from build123d import *

# Parameters (mm, degrees)
BOSS_EXTRUDE1_DEPTH                              = 10
CBORE_FOR_1_4_SOCKET_HEAD_CAP_SCREW1_D           = 7.14248
CBORE_FOR_1_4_SOCKET_HEAD_CAP_SCREW1_CBORE_D     = 11.1125
CBORE_FOR_1_4_SOCKET_HEAD_CAP_SCREW1_CBORE_DEPTH = 6.35
SKETCH5_W                                        = 12.7
SKETCH5_H                                        = 2
BOSS_EXTRUDE2_DEPTH                              = 14
CUT_EXTRUDE1_DEPTH                               = 10
SKETCH7_R                                        = 4
CUT_EXTRUDE2_DEPTH                               = 10


with BuildPart() as part:
    # Sketch1 → Boss-Extrude1 (new body)
    with BuildSketch(Plane(origin=(0, 0, 0), x_dir=(1, 0, 0), z_dir=(0, 1, 0))):
        with BuildLine():
            Line((6.35, 12.7), (6.35, -12.7))
            ThreePointArc((6.35, -12.7), (0, -19.05), (-6.35, -12.7))
            Line((-6.35, -12.7), (-6.35, 12.7))
            ThreePointArc((-6.35, 12.7), (0, 19.05), (6.35, 12.7))
        make_face()
    extrude(amount=BOSS_EXTRUDE1_DEPTH)

    # CBORE for 1/4 Socket Head Cap Screw1 (through all)
    with Locations(Plane(origin=(0, 10, 0), x_dir=(1, 0, 0), z_dir=(0, 1, 0))):
        with Locations((0, -12.7)):
            CounterBoreHole(CBORE_FOR_1_4_SOCKET_HEAD_CAP_SCREW1_D / 2, CBORE_FOR_1_4_SOCKET_HEAD_CAP_SCREW1_CBORE_D / 2, CBORE_FOR_1_4_SOCKET_HEAD_CAP_SCREW1_CBORE_DEPTH)

    # Sketch5 → Boss-Extrude2 (add)
    with BuildSketch(Plane(origin=(0, 10, 0), x_dir=(1, 0, 0), z_dir=(0, 1, 0))):
        Rectangle(SKETCH5_W, SKETCH5_H)
    extrude(amount=BOSS_EXTRUDE2_DEPTH)

    # Sketch6 → Cut-Extrude1 (cut)
    with BuildSketch(Plane.XY.offset(1)):
        with BuildLine():
            Line((-6.35, 24), (-6.35, 17.65))
            ThreePointArc((-6.35, 17.65), (-4.490128051, 22.14012807), (2.8e-08, 24))
            Line((2.8e-08, 24), (-6.35, 24))
        make_face()
        with BuildLine():
            Line((6.35, 24), (2.8e-08, 24))
            ThreePointArc((2.8e-08, 24), (4.49012807, 22.140128051), (6.35, 17.65))
            Line((6.35, 17.65), (6.35, 24))
        make_face()
    extrude(amount=-CUT_EXTRUDE1_DEPTH, mode=Mode.SUBTRACT)

    # Sketch7 → Cut-Extrude2 (cut)
    with BuildSketch(Plane.XY.offset(1)):
        with Locations((0, 17.65)):
            Circle(SKETCH7_R)
    extrude(amount=-CUT_EXTRUDE2_DEPTH, mode=Mode.SUBTRACT)


solid = part.part
The listing builds one solid part. Answer for the finished solid, in the listing's coordinates (mm). A direction names the side the tool comes from. Coordinates: 2 decimals unless noted, no trailing zeros. Loops run counter-clockwise (first coordinate to the right, second up) from the corner with the lowest first, then second, coordinate; pieces in that order, holes last. Notation, with made-up numbers: (-24.75, -8) -> (33.25, -8) arc R22 ccw to (33.25, 11) -> close; hole circle Ø11 at (69.5, 44.5). An arc over 180 degrees is marked (long way). Write item = value, one per line. Start each with the question number.
1) A cutting plane is placed at A-A (x = -2). Give the vertices of the cut face in (y, z).
2) A cutting plane is placed at C-C (y = 16.5). Give the vertices of the cut face in (x, z).
3) Given pin 1 Ø6.5 at (x, z) = (0, 12.7) entering from -Y; pin 2 Ø6 at (x, y) = (3.5, 6) entering from +Z; pin 3 Ø6 at (x, y) = (-3.5, 14) entering from -Z; pin 4 Ø2 at (x, z) = (-0.5, -5.5) entering from -Y, each flat-ended and moving along its own axis, determine where each tip first touches the part or whether it passes through.
4) Straight lines are drawn through the part: line 1 (Z direction, x = 0, y = 0.9); line 2 (Z direction, x = 0, y = 7.25); line 3 (Z direction, x = 3, y = 22). For each, find the intervals that lie inside material, in ascending order. Write a range as from..to.
5) A cutting plane is placed at B-B (z = 11). Give the vertices of the cut face in (x, y).
6) A cutting plane is placed at D-D (z = -9). Give the vertices of the cut face in (x, y).
7) The mould has two halves that part along Z. Classify faces 4 (the face through (-0.72, 6.87, 7.19)), 5 (the face through (0.46, 1.8, 9.16)), 6 (the face through (-0.14, 4.93, -19.05)), 7 (the face through (6.35, 5, 0)): released by +Z, released by -Z, zero draft, split by the parting line, or undercut.
8) A tool of negligible diameter and unlimited length cuts with its end or side. For faces 1 (the face through (-2, 14, -1)), 2 (the face through (0, 10, 6)), 3 (the face through (4, 3.65, 13)), from which of +Z, -Z, +X, -X, +Y, -Y can it reach the whole face along a straight path? Write none if from no direction.
Responses:
q1.outline = (0, -18.73) -> (10, -18.73) -> (10, -1) -> (14.19, -1) -> (14.19, 1) -> (10, 1) -> (10, 7.52) -> (3.65, 7.52) -> (3.65, 9.74) -> (0, 9.74) -> close; (0, 15.66) -> (3.65, 15.66) -> (3.65, 17.88) -> (10, 17.88) -> (10, 18.73) -> (0, 18.73) -> close; (21.11, -1) -> (23.68, -1) -> (23.68, 1) -> (21.11, 1) -> close
q2.outline = (-6.35, -1) -> (-3.83, -1) -> (-3.83, 1) -> (-6.35, 1) -> close; (3.83, -1) -> (6.35, -1) -> (6.35, 1) -> (3.83, 1) -> close
q3.pin_1 = through
q3.pin_2 = 19.03
q3.pin_3 = -1
q3.pin_4 = 0
q4.line_1 = -19.05..9.13, 16.27..19.05
q4.line_2 = -19.05..7.14, 18.26..19.05
q4.line_3 = -1..1
q5.outline = (-6.35, 0) -> (-3.14, 0) -> (-3.14, 3.65) -> (-5.29, 3.65) -> (-5.29, 10) -> (-6.35, 10) -> close; (3.14, 0) -> (6.35, 0) -> (6.35, 10) -> (5.29, 10) -> (5.29, 3.65) -> (3.14, 3.65) -> close
q6.outline = (-6.35, 0) -> (6.35, 0) -> (6.35, 10) -> (-6.35, 10) -> close
q7.face_4 = undercut
q7.face_5 = undercut
q7.face_6 = released by -Z
q7.face_7 = zero draft
q8.face_1 = -Z, +X, -X, +Y
q8.face_2 = +Z, +X, -X, +Y
q8.face_3 = +Y
